Can you work these out from the model? Positions are in its coordinate system, mm. Face numbers are marked on the shaded views. A direction names the side the tool comes from. Coordinates: 2 decimals unless noted, no trailing zeros. Order: outer loops, then holes, each group sorted by start corner. A loop starts at its lowest first (then second) coordinate and runs counter-clockwise, first axis right, second up. Notation, with made-up numbers: (37.5, 65) -> (64.5, 65) arc R21 cw to (64.5, 96) -> close; hole circle Ø9 at (14.25, 27). An arc over 180 degrees is marked (long way). Answer as CSV lines item,"result".
from build123d import *

# Parameters (mm, degrees)
F1_DEPTH = 25.4
F2_DEPTH = 25.4
F3_DEPTH = 25.4
F4_DEPTH = 25.4
F5_DEPTH = 25.4
F6_DEPTH = 25.4
F7_DEPTH = 25.4
F8_T     = -2.54


with BuildPart() as f1:
    # F0 (on Top) → F1 (new body)
    with BuildSketch(Plane.XY):
        Polygon((-27.3028922139, 0.6597405798), (-19.3204942288, 17.2683493668), (-22.6248939091, 35.3969319419), (-35.9539228893, 48.1209859294), (-54.216345136, 50.5803551806), (-70.4365360679, 41.8356442326), (-78.418934053, 25.2270354456), (-75.1145343727, 7.0984528704), (-61.7855053925, -5.625601117), (-43.5230831457, -8.0849703683), align=None)
    extrude(amount=F1_DEPTH)

    # F2 (add): a face of the model
    f2_faces = [f1.faces().sort_by_distance(p)[0] for p in [
        (-23.3116932213, 8.9640449733, 12.7),
    ]]
    extrude(f2_faces, amount=F2_DEPTH)

    # F3 (add): a face of the model
    f3_faces = [f1.faces().sort_by_distance(p)[0] for p in [
        (-74.4277350605, 33.5313398391, 12.7),
    ]]
    extrude(f3_faces, amount=F3_DEPTH)

    # F4 (add): a face of the model
    f4_faces = [f1.faces().sort_by_distance(p)[0] for p in [
        (-68.4500198826, 0.7364258767, 12.7),
    ]]
    extrude(f4_faces, amount=F4_DEPTH)

    # F5 (add): a face of the model
    f5_faces = [f1.faces().sort_by_distance(p)[0] for p in [
        (-45.0851340127, 49.350670555, 12.7),
    ]]
    extrude(f5_faces, amount=F5_DEPTH)

    # F6 (add): a face of the model
    f6_faces = [f1.faces().sort_by_distance(p)[0] for p in [
        (-7.8739129687, 11.7669152395, 12.7),
    ]]
    extrude(f6_faces, amount=F6_DEPTH)

    # F7 (add): a face of the model
    f7_faces = [f1.faces().sort_by_distance(p)[0] for p in [
        (-15.8563109538, -4.8416935475, 12.7),
    ]]
    extrude(f7_faces, amount=F7_DEPTH)

    # F8
    f8_openings = [f1.faces().sort_by_distance(p)[0] for p in [
        (-42.455515, 18.164912, 0),
    ]]
    offset(amount=F8_T, openings=f8_openings, kind=Kind.INTERSECTION)


solid = f1.part
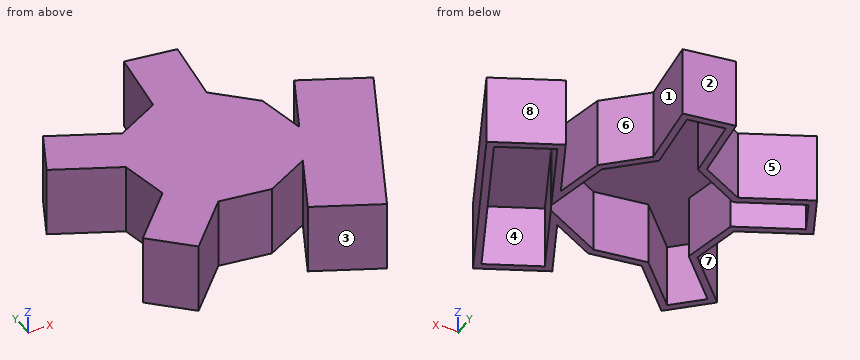
Q1. Imagine slicing it at C-C (x = 0). List the corners of the cut face in (y, z) for me.
Solution:
outline,"(-1.17, 0) -> (4.7, 0) -> (4.7, 22.86) -> (33.35, 22.86) -> (33.35, 0) -> (36.16, 0) -> (36.16, 25.4) -> (-1.17, 25.4) -> close"
Q2. Imagine slicing it at A-A (y = 20). List the corners of the cut face in (x, z) for me, and give its area (3 significant figures).
Solution:
outline,"(-77.47, 0) -> (-74.88, 0) -> (-74.88, 22.86) -> (-22.4, 22.86) -> (-22.4, 0) -> (-19.82, 0) -> (-19.82, 25.4) -> (-77.47, 25.4) -> close; (-18.01, 0) -> (-15.19, 0) -> (-15.19, 22.86) -> (7.36, 22.86) -> (7.36, 0) -> (10.17, 0) -> (10.17, 25.4) -> (-18.01, 25.4) -> close"
area,"465 mm2"
Q3. Imagine slicing it at B-B (x = -29). List the corners of the cut face in (y, z) for me.
Solution:
outline,"(-26.71, 0) -> (-23.89, 0) -> (-23.89, 22.86) -> (-8.73, 22.86) -> (-8.73, 0) -> (-2.87, 0) -> (-2.87, 25.4) -> (-26.71, 25.4) -> close; (-0.26, 0) -> (2.63, 0) -> (2.63, 22.86) -> (37.97, 22.86) -> (37.97, 0) -> (41.48, 0) -> (41.48, 25.4) -> (-0.26, 25.4) -> close"
Q4. Imagine slicing it at D-D (x = -66). List the corners of the cut face in (y, z) for me.
Solution:
outline,"(-10.04, 0) -> (-6.36, 0) -> (-6.36, 22.86) -> (41.34, 22.86) -> (41.34, 0) -> (44.23, 0) -> (44.23, 25.4) -> (-10.04, 25.4) -> close"
Q5. We'd pull the mould along Y, two halves only. Please class the marked faces 1, 2 and 3: pulls with the +Y half, pulls with the -Y half, needs draft (parallel to the pull), parting line crosses it, or undercut.
Solution:
face 1,"undercut"
face 2,"pulls with the +Y half"
face 3,"pulls with the -Y half"
Q6. If I drill on line 1 (Y direction, x = -25, z = 12.5); line 2 (X direction, y = -13.5, z = 17.75); line 3 (Y direction, x = -27, z = 10), over which ranges is the centre line in solid material (lowest first)?
Solution:
line 1,"-28.63 to -25.81, -0.41 to 4.79, 34.15 to 37.66"
line 2,"-90.32 to -86.64, -72.81 to -69.3, -34.11 to -31.29, -8.75 to -5.93"
line 3,"-27.67 to -24.85, -4.57 to 3.71, 36.06 to 39.57"
Q7. For P1, Ø1, axis at y = 26.5, z = 16.5, coming from the -X side; P2, Ø6, axis at x = -84, y = 1, coming from the -Z side; P3, Ø2, axis at x = -1, z = 6.5, coming from the +Y side; P4, Ø12, axis at y = 18.5, z = 6.5, coming from the +X side, each with a flat end and sliding along its axis, tell me the tip position at first contact or that it passes through.
Solution:
P1,"x = -82.11"
P2,"z = 0"
P3,"y = 37.13"
P4,"x = 12.34"
Q8. Which directions (+Z, -Z, +X, -X, +Y, -Y) give clear straight access to the entire face, cutting with the end or side of a thin tool? Please do the marked faces 4, 5, 6, 7 and 8.
Solution:
face 4,"-Z"
face 5,"+Z, -Z, +Y"
face 6,"+Z, -Z"
face 7,"+Z, -Z, -X"
face 8,"+Z, -Z, +X, +Y"
